Work out the finished part from the listing and answer in its coordinate system (mm). Face numbers are marked on the shaded views. A direction names the side the tool comes from. Coordinates: 2 decimals unless noted, no trailing zeros. Order: outer loops, then holes, each group sorted by start corner. A loop starts at its lowest first (then second) coordinate and runs counter-clockwise, first axis right, second up. Notation, with made-up numbers: (87, 53) -> (107, 53) arc R20 ccw to (107, 58) -> close; hole circle Ø8 at (23.25, -17.75). An arc over 180 degrees is marked (long way). Write item = value, one per line. Start each with the question number.
Q1. The part is cut by section D-D, the plane z = 117. Determine the outline of the cut face in (x, y) (3 decimals).
Q2. Which of the six approach directions +Z, -Z, +X, -X, +Y, -Y give full straight-line access (tool end or side, diameter ignored) to the marked faces 1 and 2?
Q3. The part is cut by section C-C, the plane x = -14. Determine the outline of the cut face in (y, z) (3 decimals).
Q4. The part is cut by section B-B, the plane y = -1.75. Determine the outline of the cut face in (x, z) (3 decimals).
Q5. Straight lines are drawn through the part: L1, parallel to X at y = -4.25, z = 65; L2, parallel to X at y = -3, z = 28; L3, parallel to Y at x = -17.5, z = 59 (3 decimals). For each, find the intervals that lie inside material, in ascending order. Write a range as from..to.
Q6. A flat-ended cylindrical pin translates along its axis: pin 1 (10 mm diameter, centred on x = -40, z = 83, fed in from -Y) (3 decimals). Find the tip coordinate at first contact, or state that the pin passes through.
```python
from build123d import *

# Parameters (mm, degrees)
F1_DEPTH  = 139.7
F3_DEPTH  = 139.701
F7_R      = 3.175
F8_DEPTH  = 6.35
F9_R      = 3.175
F10_DEPTH = 6.35
F11_R     = 3.175
F12_DEPTH = 6.35
F13_R     = 2.38125
F14_DEPTH = 139.701


with BuildPart() as f1:
    # F0 (on Top) → F1 (new body)
    with BuildSketch(Plane.XY):
        with BuildLine():
            Line((0, -3.175), (0, 0))
            Line((0, 0), (-47.625, 0))
            ThreePointArc((-47.625, 0), (-49.8700640303, -5.4200640303), (-44.45, -3.175))
            Line((-44.45, -3.175), (0, -3.175))
        make_face()
    extrude(amount=F1_DEPTH)

    # F2 (on face) → F3 (cut, through all)
    with BuildSketch(Plane.XY.offset(139.7)):
        with BuildLine():
            ThreePointArc((-47.625, 0), (-49.8700640303, -5.4200640303), (-44.45, -3.175))
            ThreePointArc((-44.45, -3.175), (-45.3799359697, -0.9299359697), (-47.625, 0))
        make_face()
    extrude(amount=-F3_DEPTH, mode=Mode.SUBTRACT)

    # F7 (on mid) → F8 (join, symmetric)
    with BuildSketch(Plane.XY.offset(104.775)):
        with Locations((-47.625, -3.175)):
            Circle(F7_R)
    extrude(amount=F8_DEPTH, both=True)

    # F9 (on mid) → F10 (join, symmetric)
    with BuildSketch(Plane.XY.offset(69.85)):
        with Locations((-47.625, -3.175)):
            Circle(F9_R)
    extrude(amount=F10_DEPTH, both=True)

    # F11 (on mid) → F12 (join, symmetric)
    with BuildSketch(Plane.XY.offset(34.925)):
        with Locations((-47.625, -3.175)):
            Circle(F11_R)
    extrude(amount=F12_DEPTH, both=True)

    # F13 (on face) → F14 (cut, through all)
    with BuildSketch(Plane.XY.offset(139.7)):
        with Locations((-47.625, -3.175)):
            Circle(F13_R)
    extrude(amount=-F14_DEPTH, mode=Mode.SUBTRACT)


solid = f1.part
```
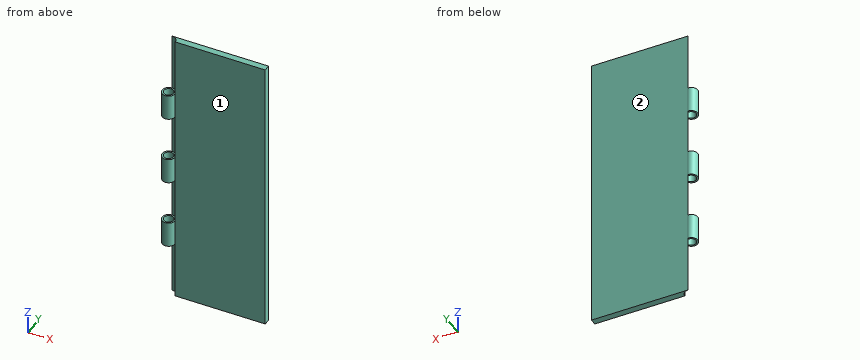
Model answer:
q1.outline = (-47.625, 0) arc R3.175 cw to (-44.45, -3.175) -> (0, -3.175) -> (0, 0) -> close
q2.face_1 = +Z, -Z, +X, -Y
q2.face_2 = +Z, -Z, +X, -X, +Y
q3.outline = (-3.175, 0) -> (0, 0) -> (0, 139.7) -> (-3.175, 139.7) -> close
q4.outline = (-50.462, 28.575) -> (-49.533, 28.575) -> (-49.533, 41.275) -> (-50.462, 41.275) -> close; (-50.462, 63.5) -> (-49.533, 63.5) -> (-49.533, 76.2) -> (-50.462, 76.2) -> close; (-50.462, 98.425) -> (-49.533, 98.425) -> (-49.533, 111.125) -> (-50.462, 111.125) -> close; (-45.717, 28.575) -> (-44.788, 28.575) -> (-44.788, 0) -> (0, 0) -> (0, 139.7) -> (-44.788, 139.7) -> (-44.788, 111.125) -> (-45.717, 111.125) -> (-45.717, 98.425) -> (-44.788, 98.425) -> (-44.788, 76.2) -> (-45.717, 76.2) -> (-45.717, 63.5) -> (-44.788, 63.5) -> (-44.788, 41.275) -> (-45.717, 41.275) -> close
q5.L1 = -50.61..-49.75, -45.5..-44.64
q5.L2 = -44.45..0
q5.L3 = -3.175..0
q6.pin_1 = -3.175
